from build123d import *

# Parameters (mm, degrees)
EXTRUDE_2_DEPTH     = 6
EXTRUDE_4_DEPTH     = 1
SKETCH_7_W          = 0.8
SKETCH_7_H          = 10
EXTRUDE_8_DEPTH     = 2.8
SKETCH_8_R          = 0.7
EXTRUDE_9_DEPTH     = 10
FILLET_1_R          = 0.85
SKETCH_11_W         = 1
SKETCH_11_H         = 1
CUT_EXTRUDE_1_DEPTH = 1.2
FILLET_2_R          = 1
SKETCH_13_W         = 0.8
SKETCH_13_H         = 10
EXTRUDE_10_DEPTH    = 1.8
SKETCH_14_R         = 0.7
EXTRUDE_11_DEPTH    = 10
FILLET_3_R          = 0.85
SKETCH_15_W         = 0.8
SKETCH_15_H         = 1
CUT_EXTRUDE_3_DEPTH = 1
FILLET_4_R          = 1
CUT_EXTRUDE_START   = -4.5
CUT_EXTRUDE_4_DEPTH = 4.5
SKETCH_17_W         = 64
SKETCH_17_H         = 25
CUT_EXTRUDE_5_DEPTH = 1.5
FILLET_5_R          = 1.5
SKETCH_20_W         = 1
SKETCH_20_H         = 0.9
EXTRUDE_14_DEPTH    = 1.5
FILLET_8_R          = 0.8
CHAMFER_3_SIZE      = 1.5


# Some blends are built 0.0001 mm under size
with BuildPart() as part:
    # case 2 → 凸台-拉伸2 (new body)
    with BuildSketch(Plane(origin=(0, 0, 0), x_dir=(1, 0, 0), z_dir=(0, 1, 0))):
        with BuildLine():
            Line((-34.042196447, 18), (30.957803553, 18))
            ThreePointArc((30.957803553, 18), (34.493337459, 16.535533906), (35.957803553, 13))
            Line((35.957803553, 13), (35.957803553, -13))
            ThreePointArc((35.957803553, -13), (34.493337459, -16.535533906), (30.957803553, -18))
            Line((30.957803553, -18), (-34.042196447, -18))
            ThreePointArc((-34.042196447, -18), (-37.577730353, -16.535533906), (-39.042196447, -13))
            Line((-39.042196447, -13), (-39.042196447, 13))
            ThreePointArc((-39.042196447, 13), (-37.577730353, 16.535533906), (-34.042196447, 18))
        make_face()
    extrude(amount=EXTRUDE_2_DEPTH)

    # 草图3 → 凸台-拉伸4 (add)
    with BuildSketch(Plane(origin=(0, 6, 0), x_dir=(1, 0, 0), z_dir=(0, 1, 0))):
        with BuildLine():
            Line((-36.892196447, 13), (-36.892196447, -13))
            ThreePointArc((-36.892196447, -13), (-35.952846076, -14.910649629), (-34.042196447, -15.85))
            Line((-34.042196447, -15.85), (30.957803553, -15.85))
            ThreePointArc((30.957803553, -15.85), (32.868453181, -14.910649629), (33.807803553, -13))
            Line((33.807803553, -13), (33.807803553, 13))
            ThreePointArc((33.807803553, 13), (32.868453181, 14.910649629), (30.957803553, 15.85))
            Line((30.957803553, 15.85), (-34.042196447, 15.85))
            ThreePointArc((-34.042196447, 15.85), (-35.952846076, 14.910649629), (-36.892196447, 13))
        make_face()
        with BuildLine():
            Line((-34.042196447, -15.05), (30.957803553, -15.05))
            ThreePointArc((30.957803553, -15.05), (32.327315928, -14.369512375), (33.007803553, -13))
            Line((33.007803553, -13), (33.007803553, 13))
            ThreePointArc((33.007803553, 13), (32.327315928, 14.369512375), (30.957803553, 15.05))
            Line((30.957803553, 15.05), (-34.042196447, 15.05))
            ThreePointArc((-34.042196447, 15.05), (-35.411708823, 14.369512375), (-36.092196447, 13))
            Line((-36.092196447, 13), (-36.092196447, -13))
            ThreePointArc((-36.092196447, -13), (-35.411708823, -14.369512375), (-34.042196447, -15.05))
        make_face(mode=Mode.SUBTRACT)
    extrude(amount=EXTRUDE_4_DEPTH)

    # 草图7 → 凸台-拉伸8 (add)
    with BuildSketch(Plane(origin=(0, 6, 0), x_dir=(1, 0, 0), z_dir=(0, 1, 0))):
        with Locations((-36.492196447, 0)):
            Rectangle(SKETCH_7_W, SKETCH_7_H)
    extrude(amount=EXTRUDE_8_DEPTH)

    # 草图8 → 凸台-拉伸9 (add)
    with BuildSketch(Plane.XY.offset(5)):
        with Locations((-36.692196447, 7.6)):
            Circle(SKETCH_8_R)
    extrude(amount=-EXTRUDE_9_DEPTH)

    # 圆角1
    # the kernel refuses this fillet: 0.85 mm, written as the material it takes off along each edge
    with BuildSketch(Plane(origin=(-36.892196447, 8.8, 6.967826014), x_dir=(0, -1, 0), z_dir=(0, 0, -1))) as fillet_1_piece_1:
        with BuildLine():
            CenterArc((0.85, -0.787130406), FILLET_1_R, 112.174937704, 67.825062296)
            Line((0, -0.787130406), (-0.017, -0.787130406))
            Line((-0.017, -0.787130406), (-0.017, 0))
            Line((-0.017, 0), (0, 0.017))
            ThreePointArc((0, 0.017), (0.264589803, 0.017), (0.522763199, 0.015742608))
            Line((0.522763199, 0.015742608), (0.529179607, 0))
        make_face()
    extrude(amount=13.935652028, mode=Mode.SUBTRACT)

    # 草图11 → 切除-拉伸1 (cut)
    with BuildSketch(Plane.ZY.offset(36.892196447)):
        with Locations((5.5, 6.5)):
            Rectangle(SKETCH_11_W, SKETCH_11_H)
        with Locations((-5.5, 6.5)):
            Rectangle(SKETCH_11_W, SKETCH_11_H)
    extrude(amount=-CUT_EXTRUDE_1_DEPTH, mode=Mode.SUBTRACT)

    # 圆角2
    fillet_2_edges = [part.edges().sort_by_distance(p)[0] for p in [
        (-36.492196447, 7, 6),
        (-36.492196447, 7, -6),
    ]]
    fillet(fillet_2_edges, radius=FILLET_2_R - 0.0001)  # a hair under: the kernel refuses the full size

    # 草图13 → 凸台-拉伸10 (add)
    with BuildSketch(Plane(origin=(0, 7, 0), x_dir=(1, 0, 0), z_dir=(0, 1, 0))):
        with Locations((33.407803553, 0)):
            Rectangle(SKETCH_13_W, SKETCH_13_H)
    extrude(amount=EXTRUDE_10_DEPTH)

    # 草图14 → 凸台-拉伸11 (add)
    with BuildSketch(Plane.XY.offset(5)):
        with Locations((33.607803553, 7.6)):
            Circle(SKETCH_14_R)
    extrude(amount=-EXTRUDE_11_DEPTH)

    # 圆角3
    # the kernel refuses this fillet: 0.85 mm, written as the material it takes off along each edge
    with BuildSketch(Plane(origin=(33.807803553, 8.8, -6.967826014), x_dir=(0, -1, 0), z_dir=(0, 0, 1))) as fillet_3_piece_1:
        with BuildLine():
            CenterArc((0.85, -0.787130406), FILLET_3_R, 112.174937704, 67.825062296)
            Line((0, -0.787130406), (-0.017, -0.787130406))
            Line((-0.017, -0.787130406), (-0.017, 0))
            Line((-0.017, 0), (0, 0.017))
            ThreePointArc((0, 0.017), (0.264589803, 0.017), (0.522763199, 0.015742608))
            Line((0.522763199, 0.015742608), (0.529179607, 0))
        make_face()
    extrude(amount=13.935652028, mode=Mode.SUBTRACT)

    # 草图15 → 切除-拉伸3 (cut)
    with BuildSketch(Plane(origin=(0, 7, 0), x_dir=(1, 0, 0), z_dir=(0, 1, 0))):
        with Locations((33.407803553, 5.5)):
            Rectangle(SKETCH_15_W, SKETCH_15_H)
        with Locations((33.407803553, -5.5)):
            Rectangle(SKETCH_15_W, SKETCH_15_H)
    extrude(amount=-CUT_EXTRUDE_3_DEPTH, mode=Mode.SUBTRACT)

    # 圆角4
    fillet_4_edges = [part.edges().sort_by_distance(p)[0] for p in [
        (33.407803553, 7, 6),
        (33.407803553, 7, -6),
    ]]
    fillet(fillet_4_edges, radius=FILLET_4_R - 0.0001)  # a hair under: the kernel refuses the full size

    # 草图16 → 切除-拉伸4 (cut)
    with BuildSketch(Plane(origin=(0, 6, 0), x_dir=(1, 0, 0), z_dir=(0, 1, 0)).offset(CUT_EXTRUDE_START)):
        with BuildLine():
            Line((-34.042196447, -15.05), (30.957803553, -15.05))
            ThreePointArc((30.957803553, -15.05), (32.327315928, -14.369512375), (33.007803553, -13))
            Line((33.007803553, -13), (33.007803553, 13))
            ThreePointArc((33.007803553, 13), (32.327315928, 14.369512375), (30.957803553, 15.05))
            Line((30.957803553, 15.05), (-34.042196447, 15.05))
            ThreePointArc((-34.042196447, 15.05), (-35.411708823, 14.369512375), (-36.092196447, 13))
            Line((-36.092196447, 13), (-36.092196447, -13))
            ThreePointArc((-36.092196447, -13), (-35.411708823, -14.369512375), (-34.042196447, -15.05))
        make_face()
    extrude(amount=CUT_EXTRUDE_4_DEPTH, mode=Mode.SUBTRACT)

    # 草图17 → 切除-拉伸5 (cut)
    with BuildSketch(Plane(origin=(0, 1.5, 0), x_dir=(1, 0, 0), z_dir=(0, 1, 0))):
        with Locations((-1.542196447, 0)):
            Rectangle(SKETCH_17_W, SKETCH_17_H)
    extrude(amount=-CUT_EXTRUDE_5_DEPTH, mode=Mode.SUBTRACT)

    # 圆角5
    fillet_5_edges = [part.edges().sort_by_distance(p)[0] for p in [
        (-33.542196447, 0.75, 12.5),
        (-33.542196447, 0.75, -12.5),
        (30.457803553, 0.75, -12.5),
        (30.457803553, 0.75, 12.5),
    ]]
    fillet(fillet_5_edges, radius=FILLET_5_R)

    # 草图20 → 凸台-拉伸14 (add)
    with BuildSketch(Plane(origin=(0, 1.5, 0), x_dir=(1, 0, 0), z_dir=(0, 1, 0))):
        with Locations((-18.542196447, 14.6)):
            Rectangle(SKETCH_20_W, SKETCH_20_H)
        with Locations((15.457803553, 14.6)):
            Rectangle(SKETCH_20_W, SKETCH_20_H)
        with Locations((-18.542196447, -14.6)):
            Rectangle(SKETCH_20_W, SKETCH_20_H)
        with Locations((15.457803553, -14.6)):
            Rectangle(SKETCH_20_W, SKETCH_20_H)
    extrude(amount=EXTRUDE_14_DEPTH)

    # 圆角8
    fillet_8_edges = [part.edges().sort_by_distance(p)[0] for p in [
        (-18.542196447, 3, -14.15),
        (15.457803553, 3, -14.15),
        (-18.542196447, 3, 14.15),
        (15.457803553, 3, 14.15),
    ]]
    fillet(fillet_8_edges, radius=FILLET_8_R)

    # 倒角3
    chamfer_3_edges = [part.edges().sort_by_distance(p)[0] for p in [
        (-1.542196447, 0, -12.5),
        (-33.102856619, 0, -12.060660172),
        (30.018463725, 0, -12.060660172),
        (-33.542196447, 0, 0),
        (30.457803553, 0, 0),
        (-33.102856619, 0, 12.060660172),
        (30.018463725, 0, 12.060660172),
        (-1.542196447, 0, 12.5),
    ]]
    chamfer(chamfer_3_edges, length=CHAMFER_3_SIZE - 0.0001)  # a hair under: the kernel refuses the full size


solid = part.part
Could you check a few things on this model? Use its own coordinates, in mm. A direction names the side the tool comes from. Give positions to 0.01 mm unless a question says otherwise; leave off trailing zeros. Order: outer loops, then holes, each group sorted by start corner. A loop starts at its lowest first (then second) coordinate and runs counter-clockwise, first axis right, second up. Notation, with made-up numbers: (66.25, 35) -> (80.25, 35) arc R31 cw to (80.25, 69) -> close; hole circle Ø6 at (71.25, 28). An arc over 180 degrees is marked (long way). Return JSON: item names as keys, results as strings.
1. Imagine slicing it at B-B on y = 5. List the corners of the cut face in (x, z) for me.
Answer list:
{"outline": "(-39.04, -13) arc R5 ccw to (-34.04, -18) -> (30.96, -18) arc R5 ccw to (35.96, -13) -> (35.96, 13) arc R5 ccw to (30.96, 18) -> (-34.04, 18) arc R5 ccw to (-39.04, 13) -> close; hole (-36.09, -13) arc R2.4 ccw to (-34.04, -15.05) -> (30.96, -15.05) arc R2.4 ccw to (33.01, -13) -> (33.01, 13) arc R2.4 ccw to (30.96, 15.05) -> (-34.04, 15.05) arc R2.4 ccw to (-36.09, 13) -> close"}
2. On a 3-axis mill with a long thin cutter (end or side, diameter ignored), from which of +Z, -Z, +X, -X, +Y, -Y can I reach the whole of each face in a straight line? I mean faces 4 (the conical face through (-33.54, 0.91, -12.46)), 5 (the cylindrical face through (-35.4, 4.21, -14.38)), 6 (the cylindrical face through (-35.931, 6.493, -14.932)), 7 (the flat face through (33.6, 7.4, 5)), 8 (the cylindrical face through (-37.616, 2.958, -16.496)). Say none if no direction works.
Answer list:
{"face 4": "-Y", "face 5": "+Y", "face 6": "-Z, -X, +Y", "face 7": "+X, -X, +Y", "face 8": "-Z, -X, +Y, -Y"}
3. I need wall thicknesses on line 1 (Z direction, x = 8.5, y = 4); line 2 (X direction, y = 5.5, z = 12); line 3 (Z direction, x = 11, y = 6.75). Which ranges of each line are inside material? Lowest first, please. Write a range as from..to.
Answer list:
{"line 1": "z = -18..-15.05, 15.05..18", "line 2": "x = -39.04..-36.09, 33.01..35.96", "line 3": "z = -15.85..-15.05, 15.05..15.85"}
4. For pin 1 Ø1.5 at (x, y) = (-36.5, 8) entering from +Z; pin 2 Ø9.5 at (x, z) = (-5, 12) entering from +Y; pin 3 Ø0.8 at (y, z) = (6.5, 10) entering from +X, each with a flat end and sliding along its axis, tell me the tip position at first contact or that it passes through.
Answer list:
{"pin 1": "stops at z = 5", "pin 2": "stops at y = 7", "pin 3": "stops at x = 33.81"}
5. Thinking about a two-plate mould opening in X: for faces 1 (the cylindrical face through (32.89, 6.49, -14.89)), 2 (the flat face through (-34.3, 0.74, 0.15)), 3 (the flat face through (1, 6, 16)), which applies, pulls with the +X half, pulls with the -X half, needs draft (parallel to the pull), parting line crosses it, or undercut?
Answer list:
{"face 1": "pulls with the +X half", "face 2": "undercut", "face 3": "needs draft"}
